from build123d import *

# Parameters (mm, degrees)
SKETCH1_W           = 90
SKETCH1_H           = 30
BOSS_EXTRUDE1_DEPTH = 4
SKETCH6_R           = 1.575
CUT_EXTRUDE6_DEPTH  = 48.602520942
SKETCH7_R           = 1.575
CUT_EXTRUDE7_DEPTH  = 48.602520942
SKETCH13_R          = 1.25
CUT_EXTRUDE13_DEPTH = 48.602520942
SKETCH14_R          = 1.25
CUT_EXTRUDE14_DEPTH = 48.602520942
FILLET1_R           = 10


with BuildPart() as part:
    # Sketch1 → Boss-Extrude1 (new body)
    with BuildSketch(Plane(origin=(0, 0, 0), x_dir=(0, 0, -1), z_dir=(1, 0, 0))):
        Rectangle(SKETCH1_W, SKETCH1_H)
    extrude(amount=BOSS_EXTRUDE1_DEPTH)

    # Sketch6 → Cut-Extrude6 (cut, through all)
    with BuildSketch(Plane(origin=(4, 0, 0), x_dir=(0, 0, -1), z_dir=(1, 0, 0))):
        with Locations((-4.75, 0)):
            Circle(SKETCH6_R)
    extrude(amount=-CUT_EXTRUDE6_DEPTH, mode=Mode.SUBTRACT)

    # Sketch7 → Cut-Extrude7 (cut, through all)
    with BuildSketch(Plane(origin=(4, 0, 0), x_dir=(0, 0, -1), z_dir=(1, 0, 0))):
        with Locations((4.75, 0)):
            Circle(SKETCH7_R)
    extrude(amount=-CUT_EXTRUDE7_DEPTH, mode=Mode.SUBTRACT)

    # Sketch13 → Cut-Extrude13 (cut, through all)
    with BuildSketch(Plane(origin=(4, 0, 0), x_dir=(0, 0, -1), z_dir=(1, 0, 0))):
        with Locations((-30, 0)):
            Circle(SKETCH13_R)
    extrude(amount=-CUT_EXTRUDE13_DEPTH, mode=Mode.SUBTRACT)

    # Sketch14 → Cut-Extrude14 (cut, through all)
    with BuildSketch(Plane(origin=(4, 0, 0), x_dir=(0, 0, -1), z_dir=(1, 0, 0))):
        with Locations((30, 0)):
            Circle(SKETCH14_R)
    extrude(amount=-CUT_EXTRUDE14_DEPTH, mode=Mode.SUBTRACT)

    # Fillet1
    fillet1_edges = [part.edges().sort_by_distance(p)[0] for p in [
        (2, -15, -45),
        (2, -15, 45),
        (2, 15, 45),
        (2, 15, -45),
    ]]
    fillet(fillet1_edges, radius=FILLET1_R)


solid = part.part
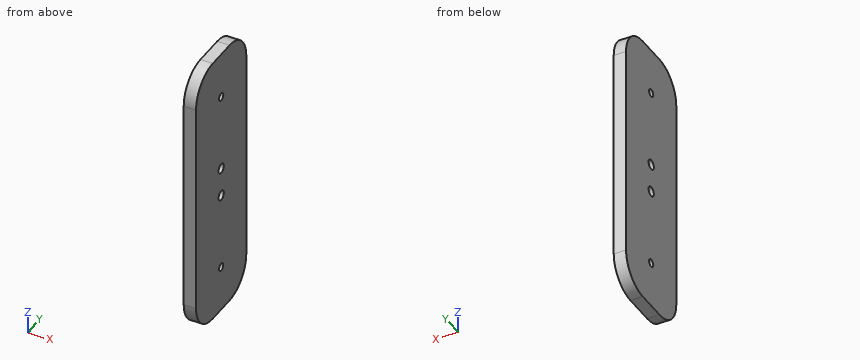
Source: CAD feature listing. Evaluate the final solid. Frame: model axes, mm. Give positions to 0.01 mm unless a question says otherwise; leave off trailing zeros. Order: outer loops, then holes, each group sorted by start corner. A loop starts at its lowest first (then second) coordinate and runs counter-clockwise, first axis right, second up. Notation, with made-up numbers: (4.5, -2) -> (58.5, -2) arc R16 cw to (58.5, 19) -> close; hole circle Ø7 at (45.5, 12). An arc over 180 degrees is marked (long way). Use a Markdown table: item, result.
1) Section query C-C, the plane z = -4.75. Return the cut outline in (x, y) (3 decimals), then the cut area to 3 significant figures.
Answer list:
| item | result |
|---|---|
| outline | (0, -15) -> (4, -15) -> (4, -1.575) -> (0, -1.575) -> close; (0, 1.575) -> (4, 1.575) -> (4, 15) -> (0, 15) -> close |
| area | 107 mm² |
2) Section query A-A, the plane x = 2.15. Return the cut outline in (y, z) (3 decimals), then the cut area to 3 significant figures.
Answer list:
| item | result |
|---|---|
| outline | (-15, -35) arc R10 ccw to (-5, -45) -> (5, -45) arc R10 ccw to (15, -35) -> (15, 35) arc R10 ccw to (5, 45) -> (-5, 45) arc R10 ccw to (-15, 35) -> close; hole circle Ø3.15 at (0, -4.75); hole circle Ø3.15 at (0, 4.75); hole circle Ø2.5 at (0, -30); hole circle Ø2.5 at (0, 30) |
| area | 2,590 mm² |
3) Section query B-B, the plane z = -30. Return the cut outline in (x, y).
Answer list:
| item | result |
|---|---|
| outline | (0, -15) -> (4, -15) -> (4, -1.25) -> (0, -1.25) -> close; (0, 1.25) -> (4, 1.25) -> (4, 15) -> (0, 15) -> close |
4) Section query D-D, the plane y = 11.5. Return the cut outline in (x, z).
Answer list:
| item | result |
|---|---|
| outline | (0, -42.6) -> (4, -42.6) -> (4, 42.6) -> (0, 42.6) -> close |
5) Ray query, line 1 along Y through (x, z) = (3.05, 30); line 2 along Z through (x, y) = (2.4, -1); line 3 along Y through (x, z) = (2.4, -4.75) (3 decimals). Return the intervals inside material, ascending. Write a range as [from, to].
Answer list:
| item | result |
|---|---|
| line 1 | [-15, -1.25], [1.25, 15] |
| line 2 | [-45, -30.75], [-29.25, -5.97], [-3.53, 3.53], [5.97, 29.25], [30.75, 45] |
| line 3 | [-15, -1.575], [1.575, 15] |
